```python
from build123d import *

# Parameters (mm, degrees)
SKETCH1_R           = 11.5
BOSS_EXTRUDE1_DEPTH = 7.9


with BuildPart() as part:
    # Sketch1 → Boss-Extrude1 (new, symmetric)
    with BuildSketch(Plane(origin=(0, 0, 0), x_dir=(1, 0, 0), z_dir=(0, 1, 0))):
        Polygon((-320, 65), (-305, 80), (305, 80), (320, 65), (320, -65), (305, -80), (-305, -80), (-320, -65), align=None)
        with Locations(Location((-220, -20, 0), (0, 0, 270))):
            Circle(SKETCH1_R, mode=Mode.SUBTRACT)
        with Locations(Location((220, -20, 0), (0, 0, 270))):
            Circle(SKETCH1_R, mode=Mode.SUBTRACT)
    extrude(amount=BOSS_EXTRUDE1_DEPTH, both=True)


solid = part.part
```
Verification items for the finished model (mm, model axes). Coordinates: 2 decimals unless noted, no trailing zeros. Order: outer loops, then holes, each group sorted by start corner. A loop starts at its lowest first (then second) coordinate and runs counter-clockwise, first axis right, second up. Notation, with made-up numbers: (-18.75, -21.75) -> (21.25, -21.75) arc R15 cw to (21.25, -6.75) -> close; hole circle Ø7 at (31, -19.5). An arc over 180 degrees is marked (long way). Put each result on its own line as item: value. Start each with the question number.
1) Cross-section at A-A (z = 20). Enter the section's corners in (x, y).
2) Material ranges on L1, parallel to X at y = 2, z = 20; L2, parallel to X at y = 5.5, z = 25.5; L3, parallel to Z at x = -219.5, y = 5.5, recorded low to high.
3) Go/stop test with a flat-tipped pin: pin 1 (20.5 mm diameter, centred on x = -220, z = 20, fed in from +Y). Record where the tip stops, or that it passes through.
4) Cross-section at B-B (x = 220). Enter the section's corners in (y, z).
5) Release check for a two-part mould opening along X. For faces 1 (the flat face through (-4, 0, -80)), 2 (the flat face through (320, 0, -1)), 3 (the cylindrical face through (209.8, -0.11, 25.31)), 4 (the flat face through (-312, 0, 73)) record: pulls with the +X half, pulls with the -X half, needs draft (parallel to the pull), parting line crosses it, or undercut.
Geometry check:
1. outline: (-320, -7.9) -> (-231.5, -7.9) -> (-231.5, 7.9) -> (-320, 7.9) -> close; (-208.5, -7.9) -> (208.5, -7.9) -> (208.5, 7.9) -> (-208.5, 7.9) -> close; (231.5, -7.9) -> (320, -7.9) -> (320, 7.9) -> (231.5, 7.9) -> close
2. L1: x = -320 to -231.5, -208.5 to 208.5, 231.5 to 320
2. L2: x = -320 to -230.1, -209.9 to 209.9, 230.1 to 320
2. L3: z = -80 to 8.51, 31.49 to 80
3. pin 1: passes through
4. outline: (-7.9, -80) -> (7.9, -80) -> (7.9, 8.5) -> (-7.9, 8.5) -> close; (-7.9, 31.5) -> (7.9, 31.5) -> (7.9, 80) -> (-7.9, 80) -> close
5. face 1: needs draft
5. face 2: pulls with the +X half
5. face 3: undercut
5. face 4: pulls with the -X half
